Autodesk Inventor part; units mm, degrees
ref_plane "YZ Plane" through (0, 0, 0) normal (1, 0, 0) x (0, 1, 0)
ref_plane "XZ Plane" through (0, 0, 0) normal (0, 1, 0) x (-1, 0, 0)
ref_plane "XY Plane" through (0, 0, 0) normal (0, 0, 1) x (1, 0, 0)
sketch "Sketch1" plane through (0, 0, 0) normal (0, 1, 0) x (-1, 0, 0)
  line L0 (0, 0) -> (25.4, 0)
  line L1 (25.4, 0) -> (25.4, -25.4)
  line L2 (25.4, -25.4) -> (0, -25.4)
  line L3 (0, -25.4) -> (0, 0)
  dimension "d0" = 25.4
  dimension "d1" = 25.4
extrude "Extrusion1" add sketch "Sketch1" along normal blind 37.7952
sketch "Sketch2" plane through (0, 0, 0) normal (0, -1, 0) x (1, 0, 0)
  line L0 (0, 0) -> (0, -25.4)
  line L1 (-25.4, 0) -> (0, 0)
  point P0 (-12.7, -12.7)
  point P1 (-12.7, 0)
  dimension "d4" = 12.7
  dimension "d5" = 12.7
hole "Hole1" at (-12.7, 0, -12.7) direction (0, 1, 0) diameter 4.9784 depth 19.05
sketch "Sketch3" plane through (-25.4, 0, -25.4) normal (-1, 0, 0) x (0, 0, 1)
  line L0 (0, 37.7952) -> (25.4, 37.7952)
  line L1 (0, 0) -> (0, 37.7952)
  point P0 (25.4, 0)
  point P1 (12.7, 25.0952)
  dimension "d13" = 12.7
  dimension "d14" = 12.7
hole "Hole2" at (-25.4, 25.0952, -12.7) direction (1, 0, 0) diameter 4.9784 end through all
sketch "Sketch4" plane through (0, 37.7952, 0) normal (0, 1, 0) x (1, 0, 0)
  line L0 (0, 25.4) -> (-25.4, 25.4)
  line L1 (-25.4, 25.4) -> (-25.4, 0)
  line L2 (-25.4, 0) -> (0, 0)
  line L3 (0, 0) -> (0, 25.4)
  line L4 (-4.7625, 25.4) -> (-4.7625, 0)
  line L5 (-25.4, 0) -> (0, 0)
  dimension "d22" = 4.7625
extrude "Extrusion2" cut sketch "Sketch4" against normal blind 25.4
extrude "Extrusion3" add sketch "Sketch4" against normal blind 25.4 contours L4 L2 L1 L0
sketch "Sketch6" plane through (-4.7625, 37.7952, 0) normal (1, 0, 0) x (0, 0, -1)
  line L0 (0, 0) -> (25.4, 0)
  line L1 (0, 0) -> (0, -25.4)
  point P0 (0, -37.7952)
  point P1 (12.7, -12.7)
  point P2 (12.7, 0)
  point P3 (0, -12.7)
  dimension "d28" = 12.7
  dimension "d29" = 12.7
hole "Hole3" at (-4.7625, 25.0952, -12.7) direction (-1, 0, 0) diameter 4.9784 end through all
sketch "Sketch7" plane through (0, 0, 0) normal (0, -1, 0) x (1, 0, 0)
  point P0 (0, 0)
sketch "Sketch8" plane through (0, 37.7952, 0) normal (0, 1, 0) x (1, 0, 0)
  line L0 (0, 25.4) -> (-25.4, 25.4)
  line L1 (0, 25.4) -> (0, 0)
  line L2 (-25.4, 25.4) -> (0, 25.4)
  line L3 (0, 25.4) -> (0, 0)
  line L4 (0, 0) -> (-25.4, 0)
  line L5 (-25.4, 0) -> (-25.4, 25.4)
extrude "Extrusion4" cut sketch "Sketch8" against normal blind 5.08
properties part number "DragBarLinkage3 Billet"
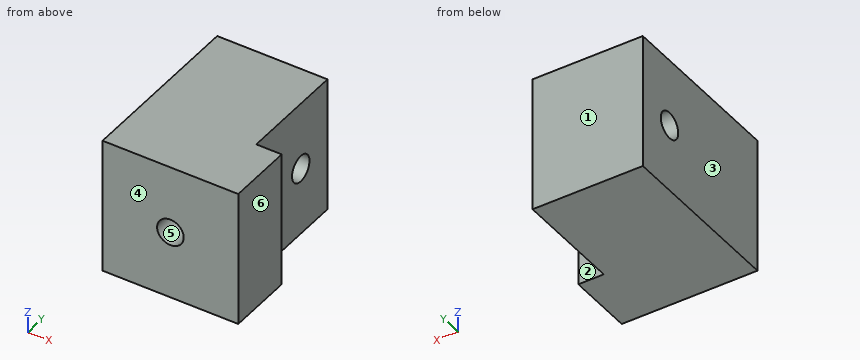
Here's how the part is built. I have some questions about the finished solid (model axes, mm). Face numbers are marked on the shaded views. A direction names the side the tool comes from. Coordinates: 2 decimals unless noted, no trailing zeros. Order: outer loops, then holes, each group sorted by start corner. A loop starts at its lowest first (then second) coordinate and runs counter-clockwise, first axis right, second up.
Item 1: If we section it at B-B on y = 8.5: List the corners of the cut face in (x, z) for me.
Result sheet:
outline: (-25.4, -25.4) - (0, -25.4) - (0, 0) - (-25.4, 0) - close; hole circle Ø4.98 at (-12.7, -12.7)
Item 2: If we section it at A-A on z = -12.7: List the corners of the cut face in (x, y) for me, plus the area to 3 significant figures.
Result sheet:
outline: (-25.4, 0) - (-15.19, 0) - (-15.19, 12.4) - (-10.21, 12.4) - (-10.21, 0) - (0, 0) - (0, 12.4) - (-4.76, 12.4) - (-4.76, 22.61) - (-25.4, 22.61) - close; (-25.4, 27.58) - (-4.76, 27.58) - (-4.76, 32.72) - (-25.4, 32.72) - close
area: 570 mm2
Item 3: If we mould it in two halves opening along X, with no side actions, what happens to the marked faces 3, 4, 5 and 6? For each: +X half, -X half, draft (parallel to the pull), parting line (faces both ways), or undercut.
Result sheet:
face 3: -X half
face 4: draft
face 5: undercut
face 6: +X half
Item 4: If we section it at D-D on z = -6.25: List the corners of the cut face in (x, y) for me, plus the area to 3 significant figures.
Result sheet:
outline: (-25.4, 0) - (0, 0) - (0, 12.4) - (-4.76, 12.4) - (-4.76, 32.72) - (-25.4, 32.72) - close
area: 734 mm2
Item 5: For the marked faces 1 and 2, which set-ups out of +Z, -Z, +X, -X, +Y, -Y let a thin tool reach every point of the face, with its end or its side?
Result sheet:
face 1: +Z, -Z, +X, -X, +Y
face 2: +Z, -Z, +X, +Y
Item 6: If we section it at C-C on x = -12.7: List the corners of the cut face in (y, z) for me.
Result sheet:
outline: (0, -25.4) - (32.72, -25.4) - (32.72, 0) - (0, 0) - (0, -10.21) - (12.4, -10.21) - (12.4, -15.19) - (0, -15.19) - close; hole circle Ø4.98 at (25.1, -12.7)
Item 7: For P1, Ø6, axis at x = -19.5, z = -19, coming from the -Y side; P2, Ø6, axis at y = 18, z = -3.5, coming from the +X side; P3, Ø4, axis at x = -2, z = -9, coming from the +Y side; P4, Ø1.5, axis at x = -13.5, z = -13, coming from the -Y side, each with a flat end and sliding along its axis, tell me the tip position at first contact or that it passes through.
Result sheet:
P1: stops at y = 0
P2: stops at x = -4.76
P3: stops at y = 12.4
P4: stops at y = 12.4
Item 8: I need wall thicknesses on line 1 (Z direction, x = -12.7, y = 8); line 2 (Y direction, x = -6.5, z = -12.5); line 3 (X direction, y = 16, z = -13.5). Which ranges of each line are inside material? Lowest first, please.
Result sheet:
line 1: z = -25.4 to -15.19, -10.21 to 0
line 2: y = 0 to 22.61, 27.58 to 32.72
line 3: x = -25.4 to -4.76
